Drawing for the job (mm, zero at the part's lowest x, y, z). A direction names the side the tool comes from. Give positions to 0.01 mm unless a question says otherwise; leave off trailing zeros. Write each loop counter-clockwise with the first axis right and the second up, starting at its lowest first coordinate (ties: lowest second). Pieces come first, ordered by that corner, then holes.
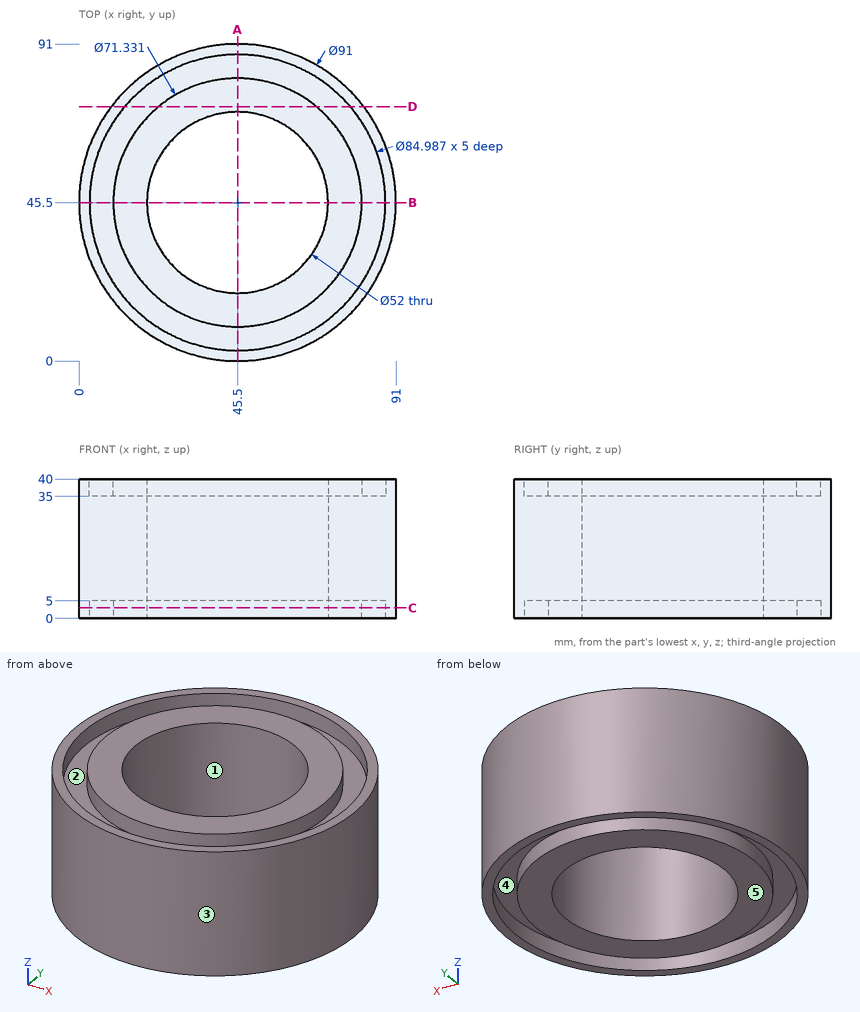
1. Slice it at D-D, the plane y = 73. Write the cut outline in (x, z) (1 decimal).
Calculated:
outline: (9.3, 0) - (13.1, 0) - (13.1, 5) - (22.8, 5) - (22.8, 0) - (68.2, 0) - (68.2, 5) - (77.9, 5) - (77.9, 0) - (81.7, 0) - (81.7, 40) - (77.9, 40) - (77.9, 35) - (68.2, 35) - (68.2, 40) - (22.8, 40) - (22.8, 35) - (13.1, 35) - (13.1, 40) - (9.3, 40) - close
2. Pin check, flat tips, straight feed: P1, Ø2, axis at y = 73.5, z = 5.5, coming from the +X side; P2, Ø3, axis at y = 37.5, z = 6.5, coming from the +X side; P3, Ø4, axis at y = 74, z = 21, coming from the -X side. Stop position of each tip, or through.
Calculated:
P1: stops at x = 82.12
P2: stops at x = 90.53
P3: stops at x = 8.51
3. Slice it at C-C, the plane z = 3. Write the cut outline in (x, y).
Calculated:
outline: circle Ø91 at (45.5, 45.5); circle Ø71.33 at (45.5, 45.5); hole circle Ø84.99 at (45.5, 45.5); hole circle Ø52 at (45.5, 45.5)
4. Probe probe 1 along Y at (x, z) = (45, 38) (1 decimal); probe 2 along X at (y, z) = (28, 37.5). List the from-to ranges inside material, lowest first.
Calculated:
probe 1: y = 0 to 3, 9.8 to 19.5, 71.5 to 81.2, 88 to 91
probe 2: x = 3.5 to 6.78, 14.42 to 26.27, 64.73 to 76.58, 84.22 to 87.5
5. Which spindle directions (+Z, -Z, +X, -X, +Y, -Y) get a long thin tool onto all of the face, cutting with end or side? Do the marked faces 1 and 2. Say none if no direction does.
Calculated:
face 1: +Z, -Z
face 2: +Z
6. Slice it at A-A, the plane x = 45.5. Write the cut outline in (y, z).
Calculated:
outline: (0, 0) - (3.01, 0) - (3.01, 5) - (9.83, 5) - (9.83, 0) - (19.5, 0) - (19.5, 40) - (9.83, 40) - (9.83, 35) - (3.01, 35) - (3.01, 40) - (0, 40) - close; (71.5, 0) - (81.17, 0) - (81.17, 5) - (87.99, 5) - (87.99, 0) - (91, 0) - (91, 40) - (87.99, 40) - (87.99, 35) - (81.17, 35) - (81.17, 40) - (71.5, 40) - close
7. Pull direction Y, two halves, no side cores. Call the marked faces 3, 4 and 5: +Y half, -Y half, draft (parallel to the pull), parting line (faces both ways), or undercut.
Calculated:
face 3: parting line
face 4: undercut
face 5: draft
